```python
from build123d import *

# Parameters (mm, degrees)
EXTRUDE_1_DEPTH = 3


with BuildPart() as part:
    # 草图1 → 凸台-拉伸1 (new body)
    with BuildSketch(Plane.XY):
        with BuildLine():
            Line((32.494506037, 1.65), (2.505493963, 1.65))
            ThreePointArc((2.505493963, 1.65), (2.87371553, 0.86125435), (3, 0))
            ThreePointArc((3, 0), (2.87371553, -0.86125435), (2.505493963, -1.65))
            Line((2.505493963, -1.65), (32.494506037, -1.65))
            ThreePointArc((32.494506037, -1.65), (32, 0), (32.494506037, 1.65))
        make_face()
        with BuildLine():
            ThreePointArc((0, -1.65), (-1.65, 0), (0, 1.65))
            Line((0, 1.65), (2.505493963, 1.65))
            ThreePointArc((2.505493963, 1.65), (-3, 0), (2.505493963, -1.65))
            Line((2.505493963, -1.65), (0, -1.65))
        make_face()
        with BuildLine():
            Line((2.505493963, 1.65), (0, 1.65))
            ThreePointArc((0, 1.65), (1.166726189, 1.166726189), (1.65, 0))
            ThreePointArc((1.65, 0), (1.166726189, -1.166726189), (0, -1.65))
            Line((0, -1.65), (2.505493963, -1.65))
            ThreePointArc((2.505493963, -1.65), (2.87371553, -0.86125435), (3, 0))
            ThreePointArc((3, 0), (2.87371553, 0.86125435), (2.505493963, 1.65))
        make_face()
        with BuildLine():
            ThreePointArc((38, 0), (35.86125435, 2.87371553), (32.494506037, 1.65))
            Line((32.494506037, 1.65), (35, 1.65))
            ThreePointArc((35, 1.65), (36.166726189, 1.166726189), (36.65, 0))
            ThreePointArc((36.65, 0), (36.166726189, -1.166726189), (35, -1.65))
            Line((35, -1.65), (32.494506037, -1.65))
            ThreePointArc((32.494506037, -1.65), (35.86125435, -2.87371553), (38, 0))
        make_face()
        with BuildLine():
            Line((35, 1.65), (32.494506037, 1.65))
            ThreePointArc((32.494506037, 1.65), (32, 0), (32.494506037, -1.65))
            Line((32.494506037, -1.65), (35, -1.65))
            ThreePointArc((35, -1.65), (33.35, 0), (35, 1.65))
        make_face()
    extrude(amount=EXTRUDE_1_DEPTH)


solid = part.part
```
Verification items for the finished model (mm, model axes). A direction names the side the tool comes from. Round coordinates to 2 decimals unless told otherwise and drop trailing zeros. Write each loop counter-clockwise with the first axis right and the second up, starting at its lowest first coordinate (ties: lowest second). Pieces come first, ordered by that corner, then holes. Notation, with made-up numbers: (-26, 21.25) - (-8, 21.25) arc R31 ccw to (-8, 59.25) - close; hole circle Ø4 at (19.25, 10.5). An arc over 180 degrees is marked (long way). Answer as a JSON object with one key per item and string values. Group by question number.
Q1. Section check C-C, the plane y = 0.5. Enter the section's corners in (x, z).
Q2. Tool access check on faces 1 (the flat face through (18, 1.65, 1)), 2 (the cylindrical face through (-3, 0, 1)). Record the directions out of +Z, -Z, +X, -X, +Y, -Y that give a thin tool (end or side, any length) a straight path to the whole face; none if there is none.
Q3. Section check D-D, the plane y = -2. Enter the section's corners in (x, z), plus the area to 3 significant figures.
Q4. Section check A-A, the plane z = 1.9. Enter the section's corners in (x, y).
Q5. Mould release check, pull along X, two halves, no side actions. Record for faces 3 (the flat face through (17, -1.65, 1)), 4 (the flat face through (17, 0, 0)): released by +X, released by -X, zero draft, split by the parting line, or undercut.
Q6. Section check B-B, the plane x = 34. Enter the section's corners in (y, z), plus the area to 3 significant figures.
Q7. Go/stop test with a flat-tipped pin: pin 1 Ø1.5 at (x, z) = (24.5, 1.5) entering from -Y. Record where the tip stops, or that it passes through.
Q8. Thickness scan on line 1 (X direction, y = 0.25, z = 2.6); line 2 (X direction, y = -1, z = 0.7); line 3 (Y direction, x = 5, z = 2). Record the ranges inside material, lowest first.
Found:
{
 "1": {"outline": "(-2.96, 0) - (-1.57, 0) - (-1.57, 3) - (-2.96, 3) - close; (1.57, 0) - (33.43, 0) - (33.43, 3) - (1.57, 3) - close; (36.57, 0) - (37.96, 0) - (37.96, 3) - (36.57, 3) - close"},
 "2": {"face 1": "+Z, -Z, +Y", "face 2": "+Z, -Z"},
 "3": {"outline": "(-2.24, 0) - (2.24, 0) - (2.24, 3) - (-2.24, 3) - close; (32.76, 0) - (37.24, 0) - (37.24, 3) - (32.76, 3) - close", "area": "26.8 mm^2"},
 "4": {"outline": "(2.51, -1.65) - (32.49, -1.65) arc R3 ccw (long way) to (32.49, 1.65) - (2.51, 1.65) arc R3 ccw (long way) to start; hole circle Ø3.3 at (0, 0); hole circle Ø3.3 at (35, 0)"},
 "5": {"face 3": "undercut", "face 4": "zero draft"},
 "6": {"outline": "(-2.83, 0) - (-1.31, 0) - (-1.31, 3) - (-2.83, 3) - close; (1.31, 0) - (2.83, 0) - (2.83, 3) - (1.31, 3) - close", "area": "9.10 mm^2"},
 "7": {"pin 1": "stops at y = -1.65"},
 "8": {"line 1": "x = -2.99 to -1.63, 1.63 to 33.37, 36.63 to 37.99", "line 2": "x = -2.83 to -1.31, 1.31 to 33.69, 36.31 to 37.83", "line 3": "y = -1.65 to 1.65"}
}
